Can you work these out from the model? Positions are in its coordinate system, mm. A direction names the side the tool comes from. Give positions to 0.01 mm unless a question says otherwise; leave off trailing zeros. Answer as a JSON object with one key per item and string values.
Autodesk Inventor part; units mm, degrees
ref_plane "YZ Plane" through (0, 0, 0) normal (1, 0, 0) x (0, 1, 0)
ref_plane "XZ Plane" through (0, 0, 0) normal (0, 1, 0) x (-1, 0, 0)
ref_plane "XY Plane" through (0, 0, 0) normal (0, 0, 1) x (1, 0, 0)
sketch "Sketch3" plane through (0, 0, 0) normal (1, 0, 0) x (0, 1, 0)
  line L0 (0, 0) -> (232.918, 0) construction
  line L1 (0, 0) -> (208.28, 0) construction
  line L2 (0, 0) -> (194.818, 0) construction
  line L3 (0, 0) -> (156.718, 0) construction
  line L4 (14.398, 96.339) -> (-14.398, -96.339) construction
  line L5 (-7.5829, 99.6241) -> (-36.3788, -93.054)
  line L6 (7.5829, -99.6241) -> (36.3788, 93.054)
  arc A0 (36.3788, 93.054) -> (-7.5829, 99.6241) centre (14.398, 96.339) ccw
  arc A1 (-36.3788, -93.054) -> (7.5829, -99.6241) centre (-14.398, -96.339) ccw
  line L7 (0, 0) -> (194.818, 0) construction
  line L8 (33.2387, 93.5233) -> (4.4428, -99.1548)
  arc A2 (-33.2387, -93.5233) -> (4.4428, -99.1548) centre (-14.398, -96.339) ccw
  line L9 (-33.2387, -93.5233) -> (-4.4428, 99.1548)
  arc A3 (33.2387, 93.5233) -> (-4.4428, 99.1548) centre (14.398, 96.339) ccw
  ellipse E0 centre (-14.398, -96.339) end of major axis (-17.2137, -115.1798) minor radius 19.05
  ellipse E1 centre (14.398, 96.339) end of major axis (33.2387, 93.5233) minor radius 19.05
  dimension "d23" = 97.409
  dimension "d24" = 98.5
  dimension "d25" = 44.45
  dimension "d26" = 3.175
extrude "Extrusion3" add sketch "Sketch3" along normal blind 127 contours A0 L6 A1 L5 | E1 A3 | A2 E0
sketch "Sketch4" plane through (127, 0, 0) normal (1, 0, 0) x (0, 0, -1)
  arc A0 (-99.1548, -4.4428) -> (-93.5233, 33.2387) centre (-96.339, 14.398) ccw
  circle A1 centre (-96.339, 14.398) radius 3.175
  line L0 (-96.339, 14.398) -> (96.339, -14.398) construction
  line L1 (-96.339, 14.398) -> (98.479, 14.398) construction
  circle A2 centre (96.339, -14.398) radius 3.175
  point P0 (0, 0)
  dimension "d27" = 6.35
  dimension "d28" = 194.818
  dimension "d29" = 8.5
  dimension "d30" = 6.35
extrude "Extrusion4" add sketch "Sketch4" along normal blind 6.35
sketch "Sketch5" plane through (133.35, 14.398, 96.339) normal (1, 0, 0) x (0, 0, -1)
  line L0 (219.7276, -97.9907) -> (219.7276, 96.8375)
  line L1 (219.7276, 96.8375) -> (-8.8724, 96.8375)
  line L2 (-8.8724, 96.8375) -> (-8.8724, -97.9907)
  line L3 (-8.8724, -97.9907) -> (219.7276, -97.9907)
  line L4 (219.7276, -97.9907) -> (414.5558, -97.9907) construction
  line L5 (-8.8724, 96.8375) -> (111.7776, 96.8375)
  line L6 (111.7776, 96.8375) -> (111.7776, 24.8285)
  line L7 (111.7776, 24.8285) -> (-8.8724, 24.8285)
  line L8 (-8.8724, 24.8285) -> (-8.8724, 96.8375)
  point P0 (96.339, -14.398)
  dimension "d33" = 90
  dimension "d34" = 228.6
  dimension "d50" = 120.65
  dimension "d51" = 72.009
extrude "Extrusion5" add sketch "Sketch5" along normal blind 3.175 contours L3 L2 L7 L6 L1 L0
sketch "Sketch6" plane through (133.35, 14.398, 96.339) normal (-1, 0, 0) x (0, 0, 1)
  line L0 (8.8724, -97.9907) -> (-219.7276, -97.9907)
  line L1 (-219.7276, -97.9907) -> (8.8724, -97.9907)
  line L2 (8.8724, -97.9907) -> (8.8724, -94.8157)
  line L3 (8.8724, -94.8157) -> (-219.7276, -94.8157)
  line L4 (-219.7276, -94.8157) -> (-219.7276, -97.9907)
  point P0 (-96.339, -14.398)
  dimension "d37" = 3.175
extrude "Extrusion6" add sketch "Sketch6" along normal blind 139.7
sketch "Sketch7" plane through (0, 0, 0) normal (-1, 0, 0) x (0, 0, 1)
  circle A0 centre (96.339, 14.398) radius 3.175
  circle A1 centre (96.339, 14.398) radius 3.175
  point P0 (0, 0)
  dimension "d40" = 6.35
extrude "Extrusion7" add sketch "Sketch7" along normal blind 6.35
sketch "Sketch8" plane through (-6.35, 14.398, 96.339) normal (-1, 0, 0) x (0, 0, 1)
  arc A0 (3.2851, -21.9809) -> (-3.2851, 21.9809) centre (0, 0) ccw construction
  line L0 (0, 0) -> (0, 25.4) construction
  line L1 (0, 25.4) -> (12.7, 25.4) construction
  line L2 (12.7, 25.4) -> (-12.7, 25.4) construction
  line L3 (-12.7, 25.4) -> (-12.7, -97.9907) construction
  line L4 (-12.7, -97.9907) -> (12.7, -97.9907) construction
  line L5 (12.7, -97.9907) -> (12.7, 25.4) construction
  line L6 (8.8724, 24.8285) -> (8.8724, -94.8157)
  line L7 (8.8724, 25.4) -> (8.8724, -97.9907)
  line L8 (8.8724, -97.9907) -> (-12.7, -97.9907)
  line L9 (-12.7, -97.9907) -> (-12.7, 25.4)
  line L10 (-111.7776, 24.8285) -> (8.8724, 24.8285)
  line L11 (-12.7, 24.8285) -> (8.8724, 24.8285)
  line L12 (-12.7, 24.8285) -> (8.8724, 24.8285) construction
  point P0 (-96.339, -14.398)
  point P1 (8.8724, 96.8375)
  point P2 (8.8724, -94.8157)
  dimension "d43" = 25.4
  dimension "d44" = 12.7
  dimension "d45" = 25.4
  dimension "d52" = 0
extrude "Extrusion8" add sketch "Sketch8" along normal blind 3.175
sketch "Sketch9" plane through (136.525, -83.5928, -123.3885) normal (0, 0, -1) x (-1, 0, 0)
  point P0 (136.525, 83.5928)
sketch "Sketch10" plane through (136.525, -83.5928, -123.3885) normal (0, 0, -1) x (-1, 0, 0)
  line L0 (142.875, 0) -> (146.05, 0)
  line L1 (142.875, 0) -> (0, 0)
  line L2 (146.05, 0) -> (0, 0)
  line L3 (0, 0) -> (0, 194.8282)
  line L4 (0, 194.8282) -> (146.05, 194.8282)
  line L5 (146.05, 194.8282) -> (146.05, 0)
  point P0 (136.525, 83.5928)
extrude "Extrusion9" add sketch "Sketch10" along normal blind 3.175
properties part number "ShootingMech_Housing5"
1) Suppose I cut it at B-B, the plane z = -69. Give the number of separate pieces and of enclosed holes in the cut face, and give its area (3 significant figures).
Answer list:
{"separate pieces": "3", "enclosed holes": "0", "area": "1,880 mm^2"}
2) Please list where these lines run through material, in increasing order: line 1 along X through (y, z) = (3, 86.5) (3 decimals); line 2 along Y through (x, z) = (113, 29); line 3 along Y through (x, z) = (39, 42.5). Write a range as from..to.
Answer list:
{"line 1": "-9.525..-6.35, 0..127, 133.35..136.525", "line 2": "-83.59..-80.42, -18.14..-14.93, 23.6..26.81", "line 3": "-83.59..-80.42, -16.12..-12.91, 25.61..28.82"}
3) For faces 1 (the flat face through (65, 15, -123.388)), 2 (the cylindrical face through (130.13, 14.26, 99.51)), 3 (the cylindrical face through (62.611, -17.199, -118.387)), which set-ups out of +Z, -Z, +X, -X, +Y, -Y let a thin tool reach every point of the face, with its end or its side?
Answer list:
{"face 1": "-X, +Y", "face 2": "none", "face 3": "-X"}
4) Will these pins go through, and if not, where does the flat tip stop? pin 1 Ø4 at (y, z) = (-2.5, -66.5) entering from -X; pin 2 Ø5 at (x, y) = (116, 54) entering from +Z; pin 3 Ø5 at (x, z) = (62, 4) entering from +Y.
Answer list:
{"pin 1": "x = 133.35", "pin 2": "z = -123.39", "pin 3": "y = 23.44"}
5) If we mould it in two halves opening along X, with no side actions, what happens to faces 4 (the flat face through (136.525, -9, -9)), 5 (the flat face through (-9.525, -21, 94)), 6 (the cylindrical face through (130.13, -15.35, -99.37)), 7 (the flat face through (65, 15, -126.564))? For each: +X half, -X half, draft (parallel to the pull), parting line (faces both ways), or undercut.
Answer list:
{"face 4": "+X half", "face 5": "-X half", "face 6": "undercut", "face 7": "draft"}
